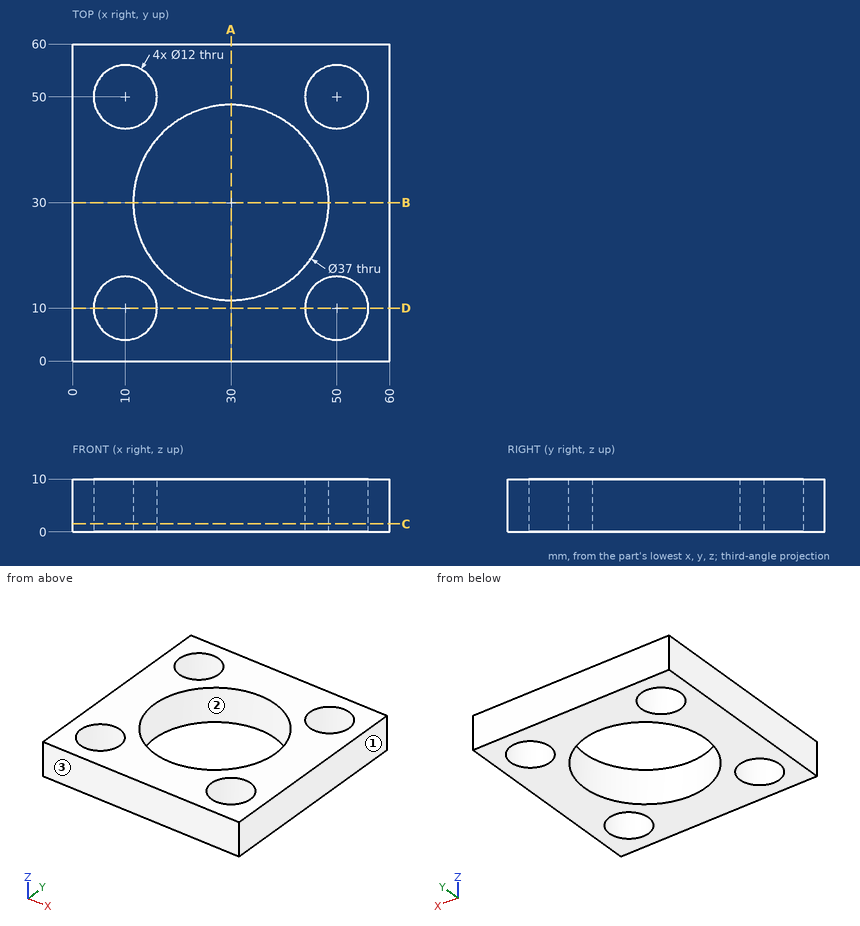
Print and shaded views of the part. All mm, measured from the part's lowest x, y and z. Give positions to 0.01 mm unless a question says otherwise; leave off trailing zeros. Order: outer loops, then holes, each group sorted by start corner. A loop starts at its lowest first (then second) coordinate and runs counter-clockwise, first axis right, second up. Notation, with made-up numbers: (33.25, -26.5) - (80.25, -26.5) arc R35 cw to (80.25, 7.5) - close; hole circle Ø1 at (65.5, 28). An arc over 180 degrees is marked (long way). One line per item, written item: value.
Item 1: Two-plate mould, pull along Y, no slides. Class the marked faces 1, 2 and 3: released by +Y, released by -Y, zero draft, split by the parting line, or undercut.
Response values:
face 1: zero draft
face 2: undercut
face 3: released by -Y
Item 2: Slice it at C-C (z = 1.5). List the corners of the cut face in (x, y).
Response values:
outline: (0, 0) - (60, 0) - (60, 60) - (0, 60) - close; hole circle Ø12 at (10, 10); hole circle Ø12 at (10, 50); hole circle Ø37 at (30, 30); hole circle Ø12 at (50, 10); hole circle Ø12 at (50, 50)
Item 3: Pin check, flat tip, straight feed: pin 1 Ø14 at (x, y) = (50, 10) entering from -Z. Stop position of the tip, or through.
Response values:
pin 1: z = 0
Item 4: Wall check: line 1 (Y direction, x = 10, z = 2.5); line 2 (X direction, y = 53.5, z = 8.5); line 3 (X direction, y = 8.5, z = 4.5). Give the ranges that are in metal, low to high.
Response values:
line 1: 0 to 4, 16 to 44, 56 to 60
line 2: 0 to 5.13, 14.87 to 45.13, 54.87 to 60
line 3: 0 to 4.19, 15.81 to 44.19, 55.81 to 60
Item 5: Slice it at D-D (y = 10). List the corners of the cut face in (x, z).
Response values:
outline: (0, 0) - (4, 0) - (4, 10) - (0, 10) - close; (16, 0) - (44, 0) - (44, 10) - (16, 10) - close; (56, 0) - (60, 0) - (60, 10) - (56, 10) - close
Item 6: Slice it at A-A (x = 30). List the corners of the cut face in (y, z).
Response values:
outline: (0, 0) - (11.5, 0) - (11.5, 10) - (0, 10) - close; (48.5, 0) - (60, 0) - (60, 10) - (48.5, 10) - close
